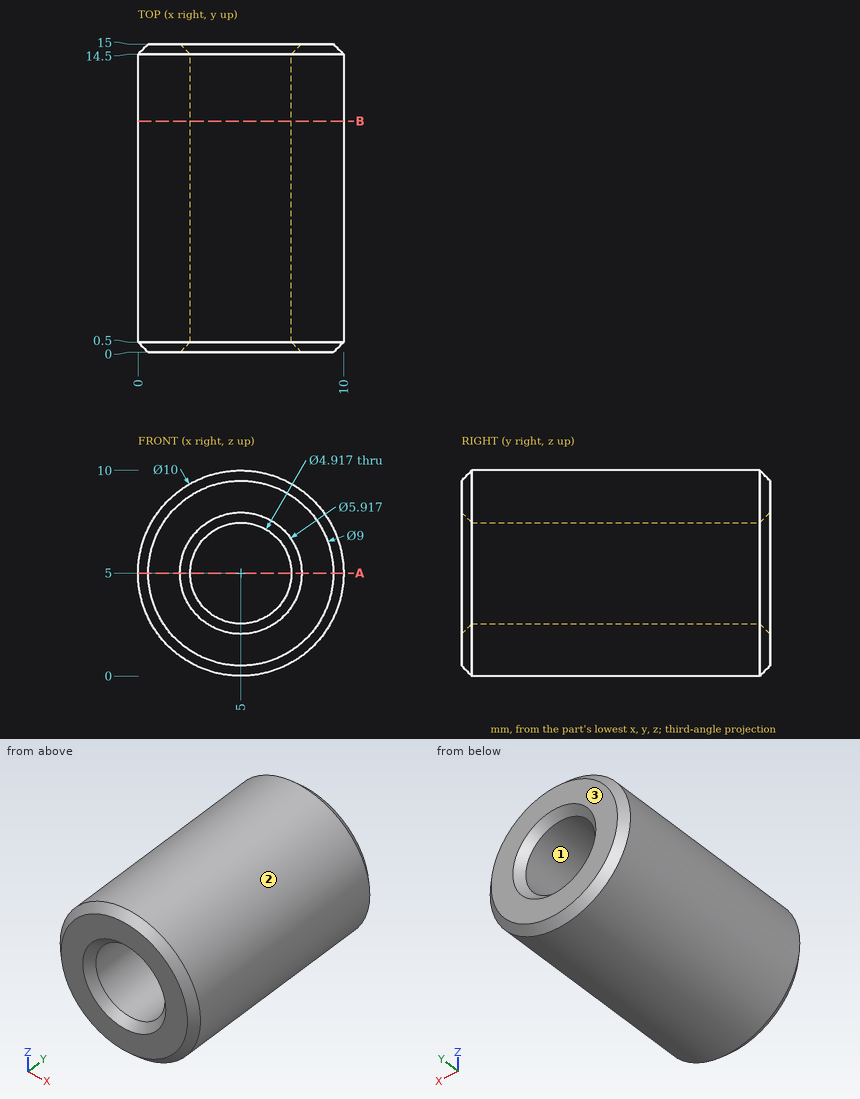
Part print with two shaded views. Sizes in mm from the minimum x, y, z corner. Round coordinates to 2 decimals unless told otherwise and drop trailing zeros. Order: outer loops, then holes, each group sorted by start corner. A loop starts at its lowest first (then second) coordinate and runs counter-clockwise, first axis right, second up. Notation, with made-up numbers: M 6,-22.75 L 49,-22.75 A33 ccw 49,7.25 Z; hole C -13,52.25 d4. An arc over 180 degrees is marked long. Put each result on its own line as item: value. Start each with the question number.
1. Two-plate mould, pull along Z, no slides. Class the marked faces 1, 2 and 3: +Z half, -Z half, draft (parallel to the pull), parting line (faces both ways), or undercut.
2. Slice it at A-A on z = 5. List the corners of the cut face in (x, y), then the cut area to 3 significant figures.
3. Drill centre lines: probe 1 along Z at (x, y) = (5, 6); probe 2 along Z at (x, y) = (4, 11.5); probe 3 along X at (y, z) = (1.5, 5.75). Where is each one in solid material? Low to high. Write a range as [from, to].
4. Drop flat-ended pins along their axis: pin 1 (5 mm diameter, centred on x = 2, y = 6, fed in from -Z); pin 2 (4 mm diameter, centred on x = 2, y = 8.5, fed in from +Z); pin 3 (6 mm diameter, centred on y = 2.5, z = 8.5, fed in from -X). Give the stop position or say it passes through.
5. Slice it at B-B on y = 11.25. List the corners of the cut face in (x, z).
Findings:
1. face 1: undercut
1. face 2: parting line
1. face 3: draft
2. outline: M 0,0.5 L 0.5,0 L 2.04,0 L 2.54,0.5 L 2.54,14.5 L 2.04,15 L 0.5,15 L 0,14.5 Z; M 7.46,0.5 L 7.96,0 L 9.5,0 L 10,0.5 L 10,14.5 L 9.5,15 L 7.96,15 L 7.46,14.5 Z
2. area: 75.2 mm2
3. probe 1: [0, 2.54], [7.46, 10]
3. probe 2: [0.1, 2.75], [7.25, 9.9]
3. probe 3: [0.06, 2.66], [7.34, 9.94]
4. pin 1: z = 0.03
4. pin 2: z = 9.9
4. pin 3: x = 0.03
5. outline: C 5,5 d10; hole C 5,5 d4.92
